from build123d import *

# Parameters (mm, degrees)
SKETCH1_W           = 66
SKETCH1_H           = 66
BOSS_EXTRUDE1_DEPTH = 2.5
SKETCH2_R           = 2
CUT_EXTRUDE1_DEPTH  = 6
SKETCH3_R           = 2
CUT_EXTRUDE2_DEPTH  = 6


with BuildPart() as part:
    # Sketch1 → Boss-Extrude1 (new body, symmetric)
    with BuildSketch(Plane.XY):
        Rectangle(SKETCH1_W, SKETCH1_H)
    extrude(amount=BOSS_EXTRUDE1_DEPTH, both=True)

    # Sketch2 → Cut-Extrude1 (cut, through all)
    with BuildSketch(Plane.XY.offset(2.5)):
        with Locations((-29, 29)):
            Circle(SKETCH2_R)
        with Locations((29, 29)):
            Circle(SKETCH2_R)
        with Locations((29, -29)):
            Circle(SKETCH2_R)
        with Locations((-29, -29)):
            Circle(SKETCH2_R)
    extrude(amount=-CUT_EXTRUDE1_DEPTH, mode=Mode.SUBTRACT)

    # Sketch3 → Cut-Extrude2 (cut, through all)
    with BuildSketch(Plane.XY.offset(2.5)):
        with Locations((0, 17.5)):
            Circle(SKETCH3_R)
        with Locations((17.5, 0)):
            Circle(SKETCH3_R)
        with Locations((0, -17.5)):
            Circle(SKETCH3_R)
        with Locations((-17.5, 0)):
            Circle(SKETCH3_R)
    extrude(amount=-CUT_EXTRUDE2_DEPTH, mode=Mode.SUBTRACT)


solid = part.part
For this review, take the finished solid that the model builds, in its own axes (mm). Give positions to 0.01 mm unless a question says otherwise; leave off trailing zeros. Loops run counter-clockwise (first coordinate to the right, second up) from the corner with the lowest first, then second, coordinate; pieces in that order, holes last. Notation, with made-up numbers: M 79,62 L 109,62 A26 ccw 109,100 Z; hole C -34,-26.5 d2. An arc over 180 degrees is marked long. Answer as a JSON object with one key per item and string values. Group by question number.
Q1. Insertion check: P1, Ø3, axis at x = 29, y = -29, coming from the +Z side. The pin has a flat end and moves straight along its axis. Give the tip position at first contact, or say it passes through.
Q2. Add section C-C on x = -17.5. Give the boundary of the cut face in (y, z), and give its area (3 significant figures).
Q3. Mouldability with a two-part tool opening along X and no side actions: class faces 1 (the cylindrical face through (-0.26, -15.517, 0.035)), 2 (the cylindrical face through (29.923, -30.774, 0.035)), 3 (the flat face through (0, -33, 0)), 4 (the flat face through (33, 0, 0)) as +X half, -X half, draft (parallel to the pull), parting line (faces both ways), or undercut.
Q4. Add section A-A on y = -29. Give the boundary of the cut face in (x, z).
Q5. For probe 1 along Y at (x, z) = (0, -1.1); probe 2 along Y at (x, z) = (-17.5, 1); probe 3 along X at (y, z) = (-18.5, 0.9), list the stretches that pass through material, from the lowest coordinate up. Write a range as [from, to].
Q6. Add section B-B on z = -1.5. Give the number of separate pieces and of enclosed holes in the cut face, and give its area (3 significant figures).
Checked values:
{
 "1": {"P1": "through"},
 "2": {"outline": "M -33,-2.5 L -2,-2.5 L -2,2.5 L -33,2.5 Z; M 2,-2.5 L 33,-2.5 L 33,2.5 L 2,2.5 Z", "area": "310 mm²"},
 "3": {"face 1": "undercut", "face 2": "undercut", "face 3": "draft", "face 4": "+X half"},
 "4": {"outline": "M -33,-2.5 L -31,-2.5 L -31,2.5 L -33,2.5 Z; M -27,-2.5 L 27,-2.5 L 27,2.5 L -27,2.5 Z; M 31,-2.5 L 33,-2.5 L 33,2.5 L 31,2.5 Z"},
 "5": {"probe 1": "[-33, -19.5], [-15.5, 15.5], [19.5, 33]", "probe 2": "[-33, -2], [2, 33]", "probe 3": "[-33, -1.73], [1.73, 33]"},
 "6": {"separate pieces": "1", "enclosed holes": "8", "area": "4,260 mm²"}
}
